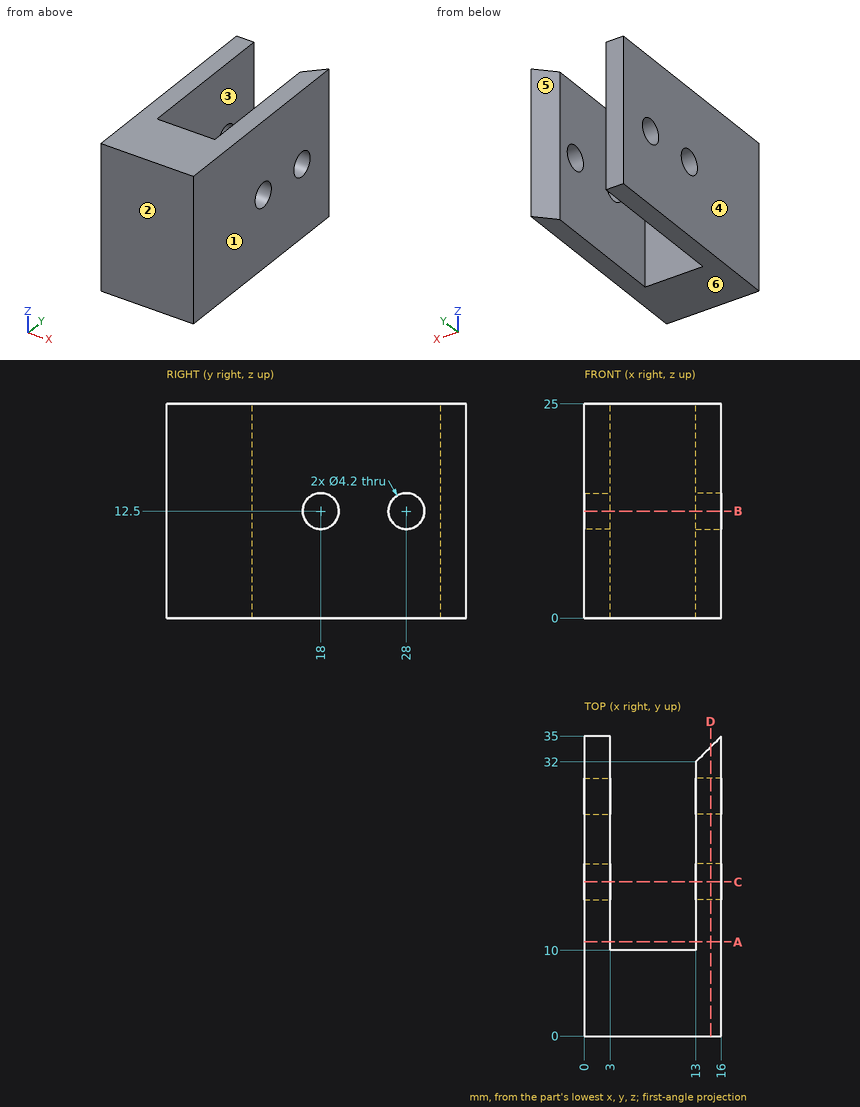
Geometry: see drawing. Coordinates: mm, zero at the bounding-box minimum. A direction names the side the tool comes from. Give positions to 0.01 mm unless a question says otherwise; leave off trailing zeros. Order: outer loops, then holes, each group sorted by start corner. A loop starts at its lowest first (then second) coordinate and runs counter-clockwise, first axis right, second up. Notation, with made-up numbers: (81.5, 68.25) -> (119.5, 68.25) arc R20 ccw to (119.5, 77.25) -> close; hole circle Ø9 at (32.25, -38.75). An arc over 180 degrees is marked (long way). Write each question's results on one line, items separated by ' | '. Start each with the question number.
1) Section B-B (z = 12.5). Return loops of the section in (x, y).
2) First-contact query: pin 1 (2 mm diameter, centred on x = 10.5, z = 9.5, fed in from -Y); pin 2 (3 mm diameter, centred on x = 7, z = 17.5, fed in from +Y). Flat tips, straight axial feed; report the tip coordinate or a pass-through.
3) Section D-D (x = 14.75). Return loops of the section in (y, z).
4) Section C-C (y = 18). Return loops of the section in (x, z), then the cut area to 3 significant figures.
5) Section A-A (y = 11). Return loops of the section in (x, z), then the cut area to 3 significant figures.
6) Set-up query: the marked faces 5 and 6. Return all of +Z, -Z, +X, -X, +Y, -Y with unobstructed straight access to the full face (end or side cutting, diameter ignored); none if empty.
7) Draft query along X for the marked faces 1, 2, 3 and 4. Return one class per face: pulls with the +X half, pulls with the -X half, needs draft (parallel to the pull), parting line crosses it, or undercut.
8) Line query: line 1 (Y direction, x = 2.3, z = 12.5); line 2 (X direction, y = 27.5, z = 21); line 3 (Z direction, x = 14.15, y = 18). Output: solid intervals per line, ascending. Write a range as from..to.
Calculated:
1) outline: (0, 0) -> (16, 0) -> (16, 15.9) -> (13, 15.9) -> (13, 10) -> (3, 10) -> (3, 15.9) -> (0, 15.9) -> close; (0, 20.1) -> (3, 20.1) -> (3, 25.9) -> (0, 25.9) -> close; (0, 30.1) -> (3, 30.1) -> (3, 35) -> (0, 35) -> close; (13, 20.1) -> (16, 20.1) -> (16, 25.9) -> (13, 25.9) -> close; (13, 30.1) -> (16, 30.1) -> (16, 35) -> (13, 32) -> close
2) pin 1: y = 0 | pin 2: y = 10
3) outline: (0, 0) -> (33.75, 0) -> (33.75, 25) -> (0, 25) -> close; hole circle Ø4.2 at (18, 12.5); hole circle Ø4.2 at (28, 12.5)
4) outline: (0, 0) -> (3, 0) -> (3, 10.4) -> (0, 10.4) -> close; (0, 14.6) -> (3, 14.6) -> (3, 25) -> (0, 25) -> close; (13, 0) -> (16, 0) -> (16, 10.4) -> (13, 10.4) -> close; (13, 14.6) -> (16, 14.6) -> (16, 25) -> (13, 25) -> close | area: 125 mm2
5) outline: (0, 0) -> (3, 0) -> (3, 25) -> (0, 25) -> close; (13, 0) -> (16, 0) -> (16, 25) -> (13, 25) -> close | area: 150 mm2
6) face 5: +Z, -Z, +Y | face 6: -Z, +X, -X, +Y, -Y
7) face 1: pulls with the +X half | face 2: needs draft | face 3: undercut | face 4: pulls with the -X half
8) line 1: 0..15.9, 20.1..25.9, 30.1..35 | line 2: 0..3, 13..16 | line 3: 0..10.4, 14.6..25
